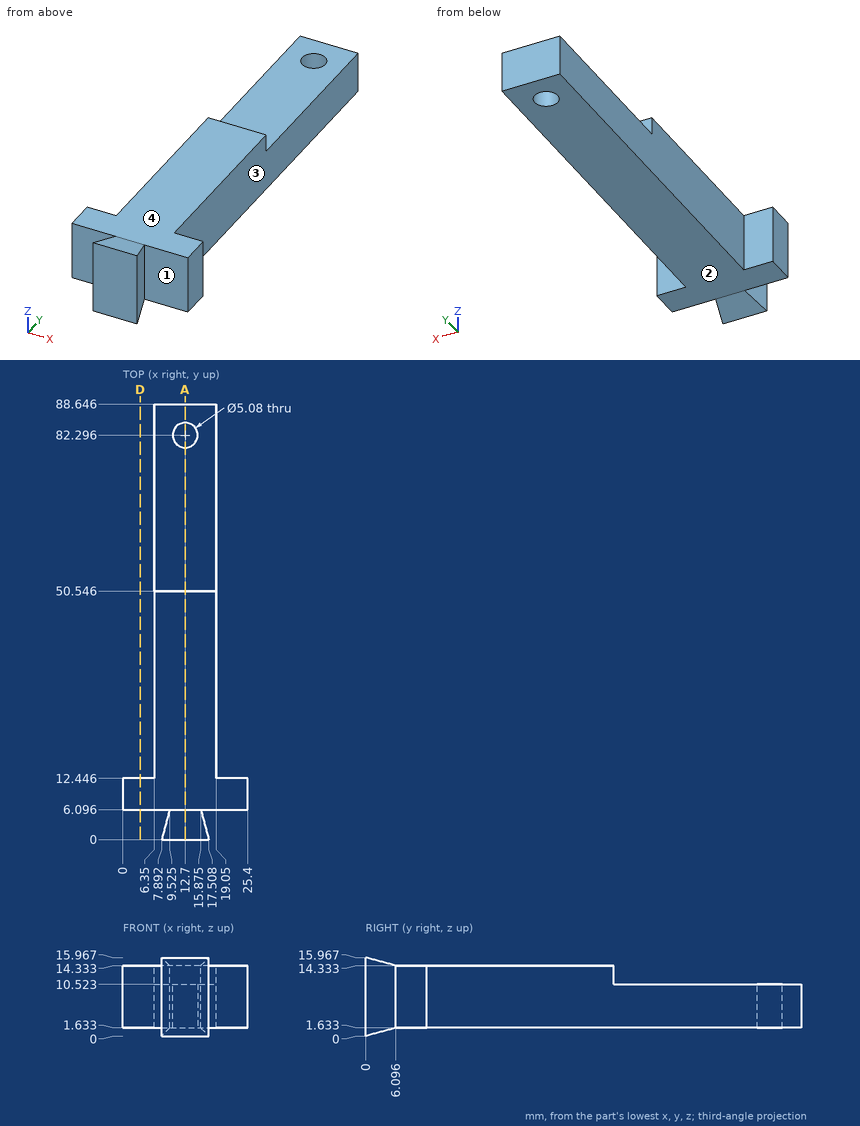
Verification items for this drawing (mm, ordinates from the low corner). A direction names the side the tool comes from. Give positions to 0.01 mm unless a question says otherwise; leave off trailing zeros. Order: outer loops, then holes, each group sorted by start corner. A loop starts at its lowest first (then second) coordinate and runs counter-clockwise, first axis right, second up.
1) Tool access check on the marked faces 1, 2, 3 and 4. Record the directions out of +Z, -Z, +X, -X, +Y, -Y that give a thin tool (end or side, any length) a straight path to the whole face; none if there is none.
Results are:
face 1: +Z, -Z, +X
face 2: -Z, +X, -X, +Y
face 3: +Z, -Z, +X, +Y
face 4: +Z, +X, -X, +Y
2) Cross-section at D-D (x = 3.5). Record the boundary of the cut face in (y, z).
Results are:
outline: (6.1, 1.63) - (12.45, 1.63) - (12.45, 14.33) - (6.1, 14.33) - close
3) Material ranges on probe 1 along Y at (x, z) = (12.7, 4); probe 2 along Y at (x, z) = (11.5, 13.75); probe 3 along X at (y, z) = (47.5, 5.75), recorded low to high.
Results are:
probe 1: y = 0 to 79.76, 84.84 to 88.65
probe 2: y = 0 to 50.55
probe 3: x = 6.35 to 19.05
4) Cross-section at A-A (x = 12.7). Record the boundary of the cut face in (y, z).
Results are:
outline: (0, 0) - (6.1, 1.63) - (79.76, 1.63) - (79.76, 10.52) - (50.55, 10.52) - (50.55, 14.33) - (6.1, 14.33) - (0, 15.97) - close; (84.84, 1.63) - (88.65, 1.63) - (88.65, 10.52) - (84.84, 10.52) - close
5) Gauge pin test, flat ends, axial feed: pin 1 (12.5 mm diameter, centred on x = 9, y = 47.5, fed in from -Z); pin 2 (4 mm diameter, centred on y = 65.5, z = 6, fed in from -X); pin 3 (5 mm diameter, centred on x = 24, z = 9, fed in from +Y). Record the tip position at first contact, or that the pin passes through.
Results are:
pin 1: stops at z = 1.63
pin 2: stops at x = 6.35
pin 3: stops at y = 12.45
